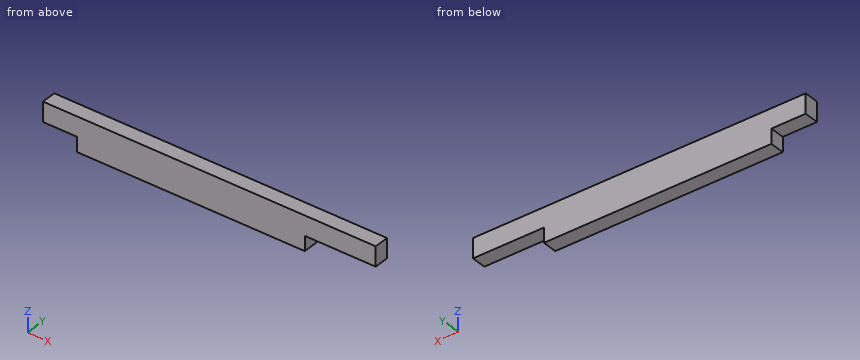
```python
from build123d import *

# Parameters (mm, degrees)
SKETCH1_W           = 863.6
SKETCH1_H           = 88.9
BOSS_EXTRUDE1_DEPTH = 38.1
SKETCH3_W           = 184.15
SKETCH3_H           = 38.1
CUT_EXTRUDE1_DEPTH  = 39.1
SKETCH4_W           = 88.9
SKETCH4_H           = 38.1
CUT_EXTRUDE2_DEPTH  = 39.1


with BuildPart() as part:
    # Sketch1 → Boss-Extrude1 (new body)
    with BuildSketch(Plane(origin=(0, 0, 0), x_dir=(1, 0, 0), z_dir=(0, 1, 0))):
        with Locations((431.8, 44.45)):
            Rectangle(SKETCH1_W, SKETCH1_H)
    extrude(amount=BOSS_EXTRUDE1_DEPTH)

    # Sketch3 → Cut-Extrude1 (cut, through all)
    with BuildSketch(Plane(origin=(0, 38.1, 0), x_dir=(1, 0, 0), z_dir=(0, 1, 0))):
        with Locations((771.525, 69.85)):
            Rectangle(SKETCH3_W, SKETCH3_H)
    extrude(amount=-CUT_EXTRUDE1_DEPTH, mode=Mode.SUBTRACT)

    # Sketch4 → Cut-Extrude2 (cut, through all)
    with BuildSketch(Plane(origin=(0, 38.1, 0), x_dir=(1, 0, 0), z_dir=(0, 1, 0))):
        with Locations((44.45, 69.85)):
            Rectangle(SKETCH4_W, SKETCH4_H)
    extrude(amount=-CUT_EXTRUDE2_DEPTH, mode=Mode.SUBTRACT)


solid = part.part
```
Geometry check sheet. Reference: the model listing, model coordinates, mm. Give positions to 0.01 mm unless a question says otherwise; leave off trailing zeros. Write each loop counter-clockwise with the first axis right and the second up, starting at its lowest first coordinate (ties: lowest second). Pieces come first, ordered by that corner, then holes.
1) Section check A-A, the plane y = 27. Record the boundary of the cut face in (x, z).
2) Material ranges on L1, parallel to X at y = 21.5, z = -69; L2, parallel to Z at x = 68.5, y = 29.5, recorded low to high.
3) Section check C-C, the plane z = -68. Record the boundary of the cut face in (x, y).
4) Gauge pin test, flat ends, axial feed: pin 1 (19 mm diameter, centred on y = 10.5, z = -73.5, fed in from -X); pin 2 (11.5 mm diameter, centred on x = 65, y = 19.5, fed in from -Z); pin 3 (1 mm diameter, centred on y = 25.5, z = -60, fed in from +X). Record the tip position at first contact, or that the pin passes through.
5) Section check B-B, the plane x = 79.5. Record the boundary of the cut face in (y, z), and give its area (3 significant figures).
Computed:
1. outline: (0, -50.8) - (88.9, -50.8) - (88.9, -88.9) - (679.45, -88.9) - (679.45, -50.8) - (863.6, -50.8) - (863.6, 0) - (0, 0) - close
2. L1: x = 88.9 to 679.45
2. L2: z = -50.8 to 0
3. outline: (88.9, 0) - (679.45, 0) - (679.45, 38.1) - (88.9, 38.1) - close
4. pin 1: stops at x = 88.9
4. pin 2: stops at z = -50.8
4. pin 3: stops at x = 679.45
5. outline: (0, -50.8) - (38.1, -50.8) - (38.1, 0) - (0, 0) - close
5. area: 1,940 mm2
